Here's how the part is built. I have some questions about the finished solid (model axes, mm). Give positions to 0.01 mm unless a question says otherwise; leave off trailing zeros. Loops run counter-clockwise (first coordinate to the right, second up) from the corner with the lowest first, then second, coordinate; pieces in that order, holes last. Notation, with made-up numbers: (-12.75, -26.5) -> (29.25, -26.5) arc R32 cw to (29.25, 5.5) -> close; hole circle Ø10 at (65.5, 35). An arc over 180 degrees is marked (long way). Answer in a Markdown table with one row per item. Add a question column.
Item 1: For P1, Ø1, axis at x = -3.5, z = 188.5, coming from the -Y side; P2, Ø1.5, axis at y = -2.5, z = 189.5, coming from the +X side; P3, Ø2, axis at y = -4.5, z = 514, coming from the +X side; P4, Ø1.5, axis at x = -0.5, z = 424, coming from the +Y side, each with a flat end and sliding along its axis, tell me the tip position at first contact or that it passes through.
Item 2: If we section it at A-A (z = 483.5): Write out the boundary of the cut face in (x, y).
Item 3: If I drill on line 1 (Y direction, x = 0, z = 21.25); line 2 (Y direction, x = 5, z = 337.5), over which ranges is the centre line in solid material (lowest first)?
```python
from build123d import *

# Parameters (mm, degrees)
CROQUIS1_R                = 6
SALIENTE_EXTRUIR1_DEPTH   = 620
TALADRO_ROSCADO_M81_D     = 6.8
TALADRO_ROSCADO_M81_DEPTH = 30
TALADRO_ROSCADO_M81_TIP   = 2.042926105
TALADRO_ROSCADO_M82_D     = 6.8
TALADRO_ROSCADO_M82_DEPTH = 30
TALADRO_ROSCADO_M82_TIP   = 2.042926105


with BuildPart() as part:
    # Croquis1 → Saliente-Extruir1 (new body)
    with BuildSketch(Plane.XY):
        Circle(CROQUIS1_R)
    extrude(amount=SALIENTE_EXTRUIR1_DEPTH)

    # Taladro roscado M81
    with Locations(Plane.XY.offset(620)):
        with Locations((0, 0)):
            Hole(TALADRO_ROSCADO_M81_D / 2, depth=TALADRO_ROSCADO_M81_DEPTH)
            with Locations((0, 0, -(TALADRO_ROSCADO_M81_DEPTH + TALADRO_ROSCADO_M81_TIP / 2))):  # 118° drill point
                Cone(0, TALADRO_ROSCADO_M81_D / 2, TALADRO_ROSCADO_M81_TIP, mode=Mode.SUBTRACT)

    # Taladro roscado M82
    with Locations(Plane(origin=(0, 0, 0), x_dir=(-1, 0, 0), z_dir=(0, 0, -1))):
        with Locations((0, 0)):
            Hole(TALADRO_ROSCADO_M82_D / 2, depth=TALADRO_ROSCADO_M82_DEPTH)
            with Locations((0, 0, -(TALADRO_ROSCADO_M82_DEPTH + TALADRO_ROSCADO_M82_TIP / 2))):  # 118° drill point
                Cone(0, TALADRO_ROSCADO_M82_D / 2, TALADRO_ROSCADO_M82_TIP, mode=Mode.SUBTRACT)


solid = part.part
```
Recorded:
| question | item | result |
|---|---|---|
| 1 | P1 | stops at y = -5.2 |
| 1 | P2 | stops at x = 5.74 |
| 1 | P3 | stops at x = 4.87 |
| 1 | P4 | stops at y = 6 |
| 2 | outline | circle Ø12 at (0, 0) |
| 3 | line 1 | y = -6 to -3.4, 3.4 to 6 |
| 3 | line 2 | y = -3.32 to 3.32 |
